from build123d import *

# Parameters (mm, degrees)
F0_R     = 1
F0_R_2   = 2.75
F0_R_3   = 9
F1_DEPTH = 3


with BuildPart() as f1:
    # F0 (on Top) → F1 (new body)
    with BuildSketch(Plane.XY):
        Polygon((0, 7), (0, 0), (20, 0), (20, 3), (30, 3), (30, 0), (50, 0), (50, 3), (55, 3), (60, 3), (60, 0), (80, 0), (80, 3), (90, 3), (90, 0), (110, 0), (110, 7), (107, 7), (107, 17), (110, 17), (110, 24), (107, 24), (107, 34), (110, 34), (110, 41), (90, 41), (90, 38), (80, 38), (80, 41), (60, 41), (60, 38), (55, 38), (50, 38), (50, 41), (30, 41), (30, 38), (20, 38), (20, 41), (0, 41), (0, 34), (3, 34), (3, 24), (0, 24), (0, 17), (3, 17), (3, 7), align=None)
        with Locations((40, 3)):
            Circle(F0_R, mode=Mode.SUBTRACT)
        with Locations((25, 12)):
            Circle(F0_R_2, mode=Mode.SUBTRACT)
        with Locations((70, 3)):
            Circle(F0_R, mode=Mode.SUBTRACT)
        with Locations((2, 20.5)):
            Circle(F0_R, mode=Mode.SUBTRACT)
        with Locations((25, 29)):
            Circle(F0_R_2, mode=Mode.SUBTRACT)
        with Locations((40, 39.5)):
            Circle(F0_R, mode=Mode.SUBTRACT)
        with Locations((90, 20.5)):
            Circle(F0_R_3, mode=Mode.SUBTRACT)
        with Locations((108, 20.5)):
            Circle(F0_R, mode=Mode.SUBTRACT)
        with Locations((70, 39.5)):
            Circle(F0_R, mode=Mode.SUBTRACT)
    extrude(amount=F1_DEPTH)


solid = f1.part
For this review, take the finished solid that the model builds, in its own axes (mm). A direction names the side the tool comes from. Coordinates: 2 decimals unless noted, no trailing zeros. Order: outer loops, then holes, each group sorted by start corner. A loop starts at its lowest first (then second) coordinate and runs counter-clockwise, first axis right, second up. Notation, with made-up numbers: (88.25, 18) -> (130.25, 18) arc R25 ccw to (130.25, 53) -> close; hole circle Ø6 at (-22, 69.25). An arc over 180 degrees is marked (long way). Return JSON: item names as keys, results as strings.
1. Machinability: for faces 1 (the cylindrical face through (69, 3, 1)), 2 (the flat face through (100, 0, 1)), 3 (the flat face through (107, 29, 1)), 4 (the flat face through (20, 1, 1)), 5 (the flat face through (55, 38, 1)), which of the approach directions +Z, -Z, +X, -X, +Y, -Y give a long, thin tool a straight path to every point of the face, cutting with its end or side? Answer none if there is none.
Answer block:
{"face 1": "+Z, -Z", "face 2": "+Z, -Z, +X, -X, -Y", "face 3": "+Z, -Z, +X", "face 4": "+Z, -Z, -Y", "face 5": "+Z, -Z, +Y"}
2. We need section B-B on x = 40. Write out the cut boundary in (y, z), and give its area (3 significant figures).
Answer block:
{"outline": "(0, 0) -> (2, 0) -> (2, 3) -> (0, 3) -> close; (4, 0) -> (38.5, 0) -> (38.5, 3) -> (4, 3) -> close; (40.5, 0) -> (41, 0) -> (41, 3) -> (40.5, 3) -> close", "area": "111 mm²"}
3. For pin 1 Ø2.5 at (x, y) = (40, 3) entering from -Z; pin 2 Ø0.9 at (x, z) = (24.5, 1.5) entering from +Y, all flat-tipped, find the tip position at first contact; note any pin that passes through.
Answer block:
{"pin 1": "z = 0", "pin 2": "y = 38"}
4. We need section A-A on y = 39.5. Write out the cut boundary in (x, z).
Answer block:
{"outline": "(0, 0) -> (20, 0) -> (20, 3) -> (0, 3) -> close; (30, 0) -> (39, 0) -> (39, 3) -> (30, 3) -> close; (41, 0) -> (50, 0) -> (50, 3) -> (41, 3) -> close; (60, 0) -> (69, 0) -> (69, 3) -> (60, 3) -> close; (71, 0) -> (80, 0) -> (80, 3) -> (71, 3) -> close; (90, 0) -> (110, 0) -> (110, 3) -> (90, 3) -> close"}
5. For line 1 (Y direction, x = 108, z = 1.35); line 2 (X direction, y = 39, z = 1.25); line 3 (X direction, y = 26.5, z = 2.5), list the stretches that pass through material, from the lowest coordinate up. Write a range as from..to.
Answer block:
{"line 1": "0..7, 17..19.5, 21.5..24, 34..41", "line 2": "0..20, 30..39.13, 40.87..50, 60..69.13, 70.87..80, 90..110", "line 3": "3..23.85, 26.15..83.29, 96.71..107"}
6. The part is to be moulded in two halves that separate along X. For faces 6 (the flat face through (1, 17, 1)), 7 (the flat face through (110, 3, 1)), 8 (the flat face through (85, 38, 1)), say which applies: +X half, -X half, draft (parallel to the pull), parting line (faces both ways), or undercut.
Answer block:
{"face 6": "draft", "face 7": "+X half", "face 8": "undercut"}
7. We need section C-C on x = 88.5. Write out the cut boundary in (y, z), and give its area (3 significant figures).
Answer block:
{"outline": "(3, 0) -> (11.63, 0) -> (11.63, 3) -> (3, 3) -> close; (29.37, 0) -> (38, 0) -> (38, 3) -> (29.37, 3) -> close", "area": "51.8 mm²"}
8. We need section D-D on x = 2. Write out the cut boundary in (y, z).
Answer block:
{"outline": "(0, 0) -> (7, 0) -> (7, 3) -> (0, 3) -> close; (17, 0) -> (19.5, 0) -> (19.5, 3) -> (17, 3) -> close; (21.5, 0) -> (24, 0) -> (24, 3) -> (21.5, 3) -> close; (34, 0) -> (41, 0) -> (41, 3) -> (34, 3) -> close"}
